from build123d import *

# Parameters (mm, degrees)
ESQUISSE1_W             = 148
ESQUISSE1_H             = 330
BOSS_EXTRU_1_DEPTH      = 3
ENL_V_MAT_EXTRU_2_REACH = 182.859
ESQUISSE3_R             = 2.2
ENL_V_MAT_EXTRU_3_REACH = 182.859
ESQUISSE4_W             = 148
ESQUISSE4_H             = 10
ENL_V_MAT_EXTRU_4_REACH = 182.859
CONG_1_SIZE             = 4
ENL_V_MAT_EXTRU_5_REACH = 182.859


with BuildPart() as part:
    # Esquisse1 → Boss.-Extru.1 (new body)
    with BuildSketch(Plane.XY):
        Rectangle(ESQUISSE1_W, ESQUISSE1_H)
    extrude(amount=BOSS_EXTRU_1_DEPTH)

    # Esquisse3 → Enl_v. mat.-Extru.2 (cut, up to next)
    with BuildSketch(Plane.XY.offset(3), mode=Mode.PRIVATE) as enl_v_mat_extru_2_sk1:
        with Locations((60, -75)):
            Circle(ESQUISSE3_R)
    enl_v_mat_extru_2_tool1 = extrude(enl_v_mat_extru_2_sk1.sketch, amount=-ENL_V_MAT_EXTRU_2_REACH, mode=Mode.PRIVATE) & part.part
    # Esquisse3 → Enl_v. mat.-Extru.2 (cut, up to next)
    with BuildSketch(Plane.XY.offset(3), mode=Mode.PRIVATE) as enl_v_mat_extru_2_sk2:
        with Locations((60, 15)):
            Circle(ESQUISSE3_R)
    enl_v_mat_extru_2_tool2 = extrude(enl_v_mat_extru_2_sk2.sketch, amount=-ENL_V_MAT_EXTRU_2_REACH, mode=Mode.PRIVATE) & part.part
    enl_v_mat_extru_2_1 = enl_v_mat_extru_2_tool1.solids().sort_by_distance((60, -75, 3))[0]
    add(enl_v_mat_extru_2_1, mode=Mode.SUBTRACT)
    enl_v_mat_extru_2_2 = enl_v_mat_extru_2_tool2.solids().sort_by_distance((60, 15, 3))[0]
    add(enl_v_mat_extru_2_2, mode=Mode.SUBTRACT)
    enl_v_mat_extru_2 = enl_v_mat_extru_2_1 + enl_v_mat_extru_2_2  # Enl_v. mat.-Extru.2 as one shape, for the pattern or mirror that repeats it

    # Esquisse4 → Enl_v. mat.-Extru.3 (cut, up to next)
    with BuildSketch(Plane.XY.offset(3), mode=Mode.PRIVATE) as enl_v_mat_extru_3_sk1:
        with Locations((0, 160)):
            Rectangle(ESQUISSE4_W, ESQUISSE4_H)
    enl_v_mat_extru_3_tool1 = extrude(enl_v_mat_extru_3_sk1.sketch, amount=-ENL_V_MAT_EXTRU_3_REACH, mode=Mode.PRIVATE) & part.part
    add(enl_v_mat_extru_3_tool1.solids().sort_by_distance((0, 160, 3))[0], mode=Mode.SUBTRACT)

    # Esquisse5 → Enl_v. mat.-Extru.4 (cut, up to next)
    with BuildSketch(Plane.XY.offset(3), mode=Mode.PRIVATE) as enl_v_mat_extru_4_sk1:
        Polygon((0, 0), (38, 0), (38, 62), (-18, 62), (-18, 0), align=None)
    enl_v_mat_extru_4_tool1 = extrude(enl_v_mat_extru_4_sk1.sketch, amount=-ENL_V_MAT_EXTRU_4_REACH, mode=Mode.PRIVATE) & part.part
    add(enl_v_mat_extru_4_tool1.solids().sort_by_distance((10, 31, 3))[0], mode=Mode.SUBTRACT)

    # Cong_1
    # a fillet whose section is not a circle: 4 mm, written as the material it adds along each edge
    with BuildSketch(Plane(origin=(38, 62, 3), x_dir=(-1, 0, 0), z_dir=(0, 0, -1)), Plane(origin=(-18, 62, 3), x_dir=(0, -1, 0), z_dir=(0, 0, -1)), Plane(origin=(38, 0, 3), x_dir=(0, 1, 0), z_dir=(0, 0, -1))) as cong_1_piece_1:
        with BuildLine():
            Bezier((CONG_1_SIZE, 0), (0, 0), (0, -CONG_1_SIZE), weights=[1, 1, 1])
            Line((0, -CONG_1_SIZE), (0, 0))
            Line((0, 0), (CONG_1_SIZE, 0))
        make_face()
    extrude(amount=3)
    with BuildSketch(Plane(origin=(-18, 0, 3), x_dir=(0, 1, 0), z_dir=(0, 0, -1))) as cong_1_piece_2:
        with BuildLine():
            Bezier((CONG_1_SIZE, 0), (0, 0), (0, CONG_1_SIZE), weights=[1, 1, 1])
            Line((0, CONG_1_SIZE), (0, 0))
            Line((0, 0), (CONG_1_SIZE, 0))
        make_face()
    extrude(amount=3)

    # Esquisse6 → Enl_v. mat.-Extru.5 (cut, up to next)
    with BuildSketch(Plane(origin=(0, 0, 0), x_dir=(-1, 0, 0), z_dir=(0, 0, -1)), mode=Mode.PRIVATE) as enl_v_mat_extru_5_sk1:
        Polygon((17, -49), (37, -49), (41, -53), (41, -73), (37, -77), (17, -77), (13, -73), (13, -53), align=None)
    enl_v_mat_extru_5_tool1 = extrude(enl_v_mat_extru_5_sk1.sketch, amount=-ENL_V_MAT_EXTRU_5_REACH, mode=Mode.PRIVATE) & part.part
    add(enl_v_mat_extru_5_tool1.solids().sort_by_distance((-27, -63, 0))[0], mode=Mode.SUBTRACT)

    # Sym_trie1: Enl_v. mat.-Extru.2 across plane
    add(enl_v_mat_extru_2.mirror(Plane(origin=(0, 0, 0), x_dir=(0, 0, 1), z_dir=(1, 0, 0))), mode=Mode.SUBTRACT)


solid = part.part
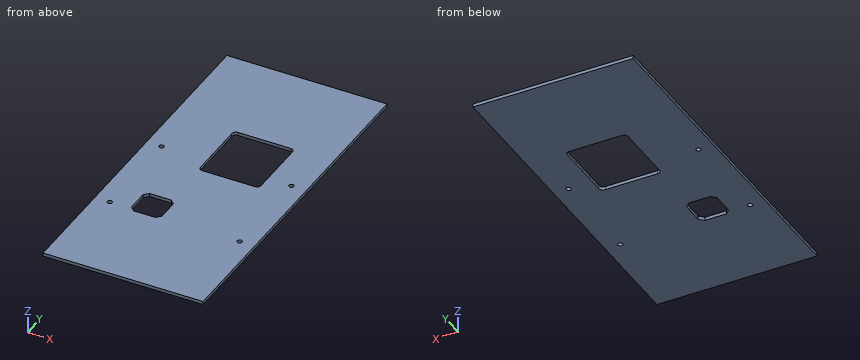
Build history of the part. All positions in model axes, mm. Coordinates: 2 decimals unless noted, no trailing zeros. Write each loop counter-clockwise with the first axis right and the second up, starting at its lowest first coordinate (ties: lowest second). Pieces come first, ordered by that corner, then holes.
(1) Cut at C-C on z = 1.1. State how many separate pieces and enclosed holes the cut face has, and give its area (3 significant figures).
(2) Cut at B-B on x = 8.5. List the corners of the cut face in (y, z).
(3) Pin check, flat tip, straight feed: pin 1 Ø2.5 at (x, y) = (60, 15) entering from -Z. Stop position of the tip, or through.
(4) Drill centre lines: line 1 (Y direction, x = -60, z = 1.9); line 2 (Y direction, x = -1, z = 0.85); line 3 (X direction, y = 29.5, z = 0.95). Where is each one in solid material? Low to high.
(5) Cut at A-A on y = 45.5. List the corners of the cut face in (x, z), and give its area (3 significant figures).
Working result:
1. separate pieces: 1
1. enclosed holes: 6
1. area: 43,100 mm2
2. outline: (-165, 0) - (0, 0) - (0, 3) - (-165, 3) - close; (62, 0) - (155, 0) - (155, 3) - (62, 3) - close
3. pin 1: passes through
4. line 1: y = -165 to -77.2, -72.8 to 12.8, 17.2 to 155
4. line 2: y = -165 to 0, 62 to 155
4. line 3: x = -74 to -18, 38 to 74
5. outline: (-74, 0) - (-18, 0) - (-18, 3) - (-74, 3) - close; (38, 0) - (74, 0) - (74, 3) - (38, 3) - close
5. area: 276 mm2
